Verification items for this drawing (mm, ordinates from the low corner). Give positions to 0.01 mm unless a question says otherwise; leave off trailing zeros. Order: outer loops, then holes, each group sorted by start corner. A loop starts at its lowest first (then second) coordinate and runs counter-clockwise, first axis right, second up. Notation, with made-up numbers: (-29.75, 45.25) -> (7.25, 45.25) arc R29 ccw to (7.25, 83.25) -> close; hole circle Ø6 at (58, -22.75). An arc over 180 degrees is marked (long way). One line per question, with ' | ' between items.
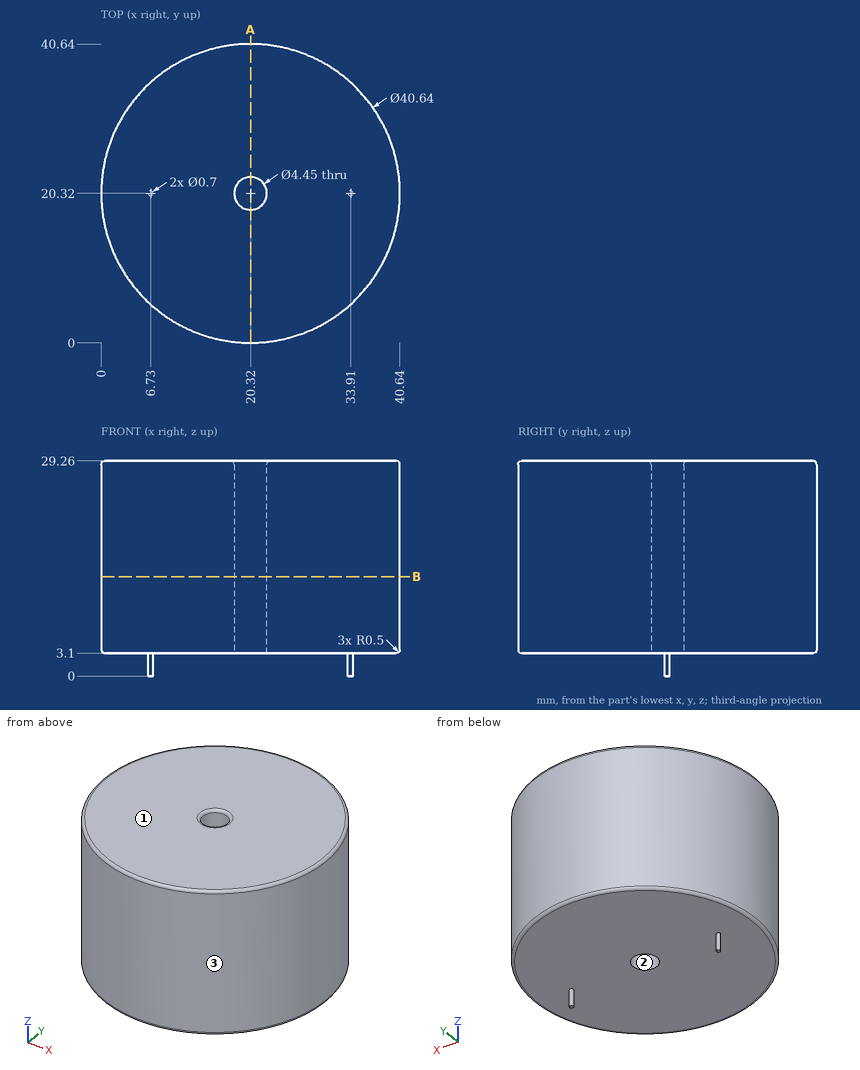
Q1. Mould release check, pull along X, two halves, no side actions. Record for the marked faces 1, 2 and 3: pulls with the +X half, pulls with the -X half, needs draft (parallel to the pull), parting line crosses it, or undercut.
Result sheet:
face 1: needs draft | face 2: undercut | face 3: parting line crosses it
Q2. Section check B-B (z = 13.5). Enter the section's corners in (x, y) (3 decimals).
Result sheet:
outline: circle Ø40.64 at (20.32, 20.32); hole circle Ø4.45 at (20.32, 20.32)
Q3. Thickness scan on line 1 (Y direction, x = 20.32, z = 16.75) (3 decimals); line 2 (Z direction, x = 12, y = 12.5); line 3 (X direction, y = 21.5, z = 15.25). Record the ranges inside material, lowest first.
Result sheet:
line 1: y = 0 to 18.095, 22.545 to 40.64 | line 2: z = 3.1 to 29.26 | line 3: x = 0.03 to 18.43, 22.21 to 40.61
Q4. Section check A-A (x = 20.32). Enter the section's corners in (y, z) (3 decimals), and give its area (3 significant figures).
Result sheet:
outline: (0, 3.6) arc R0.5 ccw to (0.5, 3.1) -> (18.095, 3.1) -> (18.095, 28.76) arc R0.5 ccw to (17.595, 29.26) -> (0.5, 29.26) arc R0.5 ccw to (0, 28.76) -> close; (22.545, 3.1) -> (40.14, 3.1) arc R0.5 ccw to (40.64, 3.6) -> (40.64, 28.76) arc R0.5 ccw to (40.14, 29.26) -> (23.045, 29.26) arc R0.5 ccw to (22.545, 28.76) -> close | area: 946 mm2
Q5. Depth check by flat-ended pin: pin 1 Ø2 at (x, z) = (24, 17.5) entering from +Y; pin 2 Ø1 at (x, z) = (11.5, 21) entering from -Y; pin 3 Ø6 at (x, z) = (23.5, 20) entering from +Y; pin 4 Ø4 at (x, y) = (20.32, 20.32) entering from +Z. Enter the tip coordinate at first touch or a pass-through.
Result sheet:
pin 1: stops at y = 40.46 | pin 2: stops at y = 1.78 | pin 3: stops at y = 40.64 | pin 4: passes through
